Autodesk Inventor part; units mm, degrees
ref_plane "YZ Plane" through (0, 0, 0) normal (1, 0, 0) x (0, 1, 0)
ref_plane "XZ Plane" through (0, 0, 0) normal (0, 1, 0) x (-1, 0, 0)
ref_plane "XY Plane" through (0, 0, 0) normal (0, 0, 1) x (1, 0, 0)
sketch "Sketch1" plane through (0, 0, 0) normal (0, 0, 1) x (1, 0, 0)
  circle A0 centre (0, 0) radius 3
  circle A1 centre (0, 0) radius 3
  circle A2 centre (0, 0) radius 4
  point P0 (0, 0)
  dimension "d0" = 6
  dimension "d1" = 8
extrude "Extrusion1" add sketch "Sketch1" against normal blind 2
ref_plane "Work Plane1" through (0, 0, -1) normal (0, 0, 1) x (1, 0, 0)
sketch "Sketch2" plane through (0, 0, 0) normal (0, 1, 0) x (-1, 0, 0)
  line L0 (4, 0) -> (4, -2)
  line L1 (4, -1) -> (3.5, -1)
  line L2 (4, -1) -> (4, -1.5)
  line L3 (4, -1) -> (4, -0.5)
  line L4 (4, -0.5) -> (3.5, -1)
  line L5 (4, -1.5) -> (3.5, -1)
  line L6 (0, 0) -> (0, -2)
  line L7 (-4, -2) -> (4, -2)
  dimension "d4" = 0.5
  dimension "d5" = 0.5
  dimension "d6" = 0.5
revolve "Revolution1" cut sketch "Sketch2" angle 360 about axis through (0, 0, 0) along (0, 0, -1)
fillet "Fillet1" radius 0.2 1 edges at (3.5, 0, -1)
properties part number "c_roller_1"
CAD build for the part. Positions are in the model's coordinates, mm. Round coordinates to 2 decimals unless told otherwise and drop trailing zeros. Write each loop counter-clockwise with the first axis right and the second up, starting at its lowest first coordinate (ties: lowest second). Pieces come first, ordered by that corner, then holes. Notation, with made-up numbers: M 30,19.5 L 63,19.5 A7 cw 63,28.5 Z; hole C -18,-20.5 d2. An arc over 180 degrees is marked long. Use a Markdown table: item, result. Add a question column.
1. Drill centre lines: probe 1 along Y at (x, z) = (0, -1.55); probe 2 along Y at (x, z) = (2.25, -1.15); probe 3 along X at (y, z) = (-1.5, -1.9). Where is each one in solid material? Low to high.
2. Pull direction Y, two halves, no side cores. Call faces 1 (the face through (-0.867, -3.905, -1.746)), 2 (the face through (1, 3, 0)), 3 (the face through (-3, 0, -1)): released by +Y, released by -Y, zero draft, split by the parting line, or undercut.
3. Flat gauge pins, fed straight in: P1, Ø1, axis at x = 1.5, z = -0.5, coming from the +Y side; P2, Ø1, axis at y = 2.5, z = -0.5, coming from the +X side. Where does each tip first touch, or does it go through?
4. Slice it at A-A on z = -0.3. Give the cut face in (x, y).
Reply:
| question | item | result |
|---|---|---|
| 1 | probe 1 | y = -4 to -3, 3 to 4 |
| 1 | probe 2 | y = -2.87 to -1.98, 1.98 to 2.87 |
| 1 | probe 3 | x = -3.71 to -2.6, 2.6 to 3.71 |
| 2 | face 1 | split by the parting line |
| 2 | face 2 | zero draft |
| 2 | face 3 | undercut |
| 3 | P1 | stops at y = 3.87 |
| 3 | P2 | stops at x = 3.46 |
| 4 | outline | C 0,0 d8; hole C 0,0 d6 |
